Could you check a few things on this model? Use its own coordinates, in mm. Face numbers are marked on the shaded views. A direction names the side the tool comes from. Round coordinates to 2 decimals unless told otherwise and drop trailing zeros. Loops run counter-clockwise (first coordinate to the right, second up) from the corner with the lowest first, then second, coordinate; pieces in that order, holes last.
from build123d import *

# Parameters (mm, degrees)
EXTRUDE_1_DEPTH              = 2
EXTRUDE_3_DEPTH              = 6
CUT_EXTRUDE_1_REACH          = 27.426
SKETCH_5_R                   = 1.25
EXTRUDE_4_REACH              = 39.53
SKETCH_6_W                   = 10
SKETCH_6_H                   = 0.5
CUT_EXTRUDE_2_REACH          = 39.53
SKETCH_7_W                   = 8
SKETCH_7_H                   = 0.5
SKETCH_10_W                  = 1
SKETCH_10_H                  = 3.5
EXTRUDE_5_DEPTH              = 3.3
CHAMFER_1_SIZE               = 2
CUT_EXTRUDE_3_REACH          = 27.114
CUT_EXTRUDE_4_DEPTH          = 0.5
HOLE_WIZARD_M2_2_D           = 2.1
HOLE_WIZARD_M2_2_CBORE_D     = 3.8
HOLE_WIZARD_M2_2_CBORE_DEPTH = 1
FILLET_3_R                   = 2
CUT_EXTRUDE_5_DEPTH          = 0.8


with BuildPart() as part:
    # ｽｹｯﾁ1 → ﾎﾞｽ - 押し出し1 (new body)
    with BuildSketch(Plane(origin=(0, 0, 0), x_dir=(1, 0, 0), z_dir=(0, 1, 0))):
        Polygon((-13, 8), (3, 8), (13, 1), (13, -8), (-13, -8), (-13, -5), (-23.5, 2.35), (-23.5, 8), align=None)
    extrude(amount=EXTRUDE_1_DEPTH)

    # ｽｹｯﾁ4 → ﾎﾞｽ - 押し出し3 (add)
    with BuildSketch(Plane.XY.offset(8)):
        Polygon((-7, -3.5), (-4.5, -3.5), (-3, 0), (-7.9, 0), align=None)
        Polygon((3, 0), (4.5, -3.5), (7, -3.5), (7.9, 0), align=None)
    extrude(amount=-EXTRUDE_3_DEPTH)

    # ｽｹｯﾁ5 → ｶｯﾄ - 押し出し1 (cut, up to next)
    with BuildSketch(Plane(origin=(0, 2, 0), x_dir=(1, 0, 0), z_dir=(0, 1, 0)), mode=Mode.PRIVATE) as cut_extrude_1_sk1:
        with Locations(Location((0, -5, 0), (0, 0, 270))):
            Circle(SKETCH_5_R)
    cut_extrude_1_tool1 = extrude(cut_extrude_1_sk1.sketch, amount=-CUT_EXTRUDE_1_REACH, mode=Mode.PRIVATE) & part.part
    add(cut_extrude_1_tool1.solids().sort_by_distance((0, 2, 5))[0], mode=Mode.SUBTRACT)

    # ﾎﾞｽ - 押し出し4: up to this face of the body (flat: up to its plane)
    extrude_4_end = Plane(part.part.faces().sort_by_distance((-23.5, 1, -5.175))[0])
    # ｽｹｯﾁ6 → ﾎﾞｽ - 押し出し4 (add, up to the picked face)
    with BuildSketch(Plane(origin=(13, 0, 0), x_dir=(0, 0, -1), z_dir=(1, 0, 0)), mode=Mode.PRIVATE) as extrude_4_sk1:
        with Locations((3, -0.25)):
            Rectangle(SKETCH_6_W, SKETCH_6_H)
    extrude_4_tool1 = split(extrude(extrude_4_sk1.sketch, amount=-EXTRUDE_4_REACH, mode=Mode.PRIVATE), bisect_by=extrude_4_end, keep=Keep.BOTH, mode=Mode.PRIVATE)
    add(extrude_4_tool1.solids().sort_by(Axis((13, -0.25, -3), (-1, 0, 0)))[0])

    # ｽｹｯﾁ7 → ｶｯﾄ - 押し出し2 (cut, up to next)
    with BuildSketch(Plane(origin=(13, 0, 0), x_dir=(0, 0, -1), z_dir=(1, 0, 0)), mode=Mode.PRIVATE) as cut_extrude_2_sk1:
        with Locations((4, 1.75)):
            Rectangle(SKETCH_7_W, SKETCH_7_H)
    cut_extrude_2_tool1 = extrude(cut_extrude_2_sk1.sketch, amount=-CUT_EXTRUDE_2_REACH, mode=Mode.PRIVATE) & part.part
    add(cut_extrude_2_tool1.solids().sort_by_distance((13, 1.75, -4))[0], mode=Mode.SUBTRACT)

    # ｽｹｯﾁ10 → ﾎﾞｽ - 押し出し5 (add)
    with BuildSketch(Plane.XZ.offset(0.5)):
        with Locations((10.75, 0.25)):
            Rectangle(SKETCH_10_W, SKETCH_10_H)
    extrude_5 = extrude(amount=EXTRUDE_5_DEPTH)

    # ﾐﾗｰ1: ﾎﾞｽ - 押し出し5 across plane
    add(extrude_5.mirror(Plane(origin=(0, 0, 0), x_dir=(0, 0, 1), z_dir=(1, 0, 0))))

    # 面取り1
    # the kernel refuses this chamfer: 2 mm, written as the material it takes off along each edge
    with BuildSketch(Plane(origin=(18.143365976, 2, 8), x_dir=(0, -0.9996219169112968, 0.027495876610586494), z_dir=(-1, 0, 0))) as chamfer_1_piece_1:
        Polygon((CHAMFER_1_SIZE * 0.999621916911, -CHAMFER_1_SIZE * 0.0274958766106), (-CHAMFER_1_SIZE * 0.0274958766106, -CHAMFER_1_SIZE * 0.999621916911), (0, 0), align=None)
    extrude(amount=36.286731952, mode=Mode.SUBTRACT)

    # ｽｹｯﾁ12 → ｶｯﾄ - 押し出し3 (cut, up to next)
    with BuildSketch(Plane(origin=(0, 0, 0), x_dir=(1, 0, 0), z_dir=(0, 1, 0)), mode=Mode.PRIVATE) as cut_extrude_3_sk1:
        Polygon((3, 8), (13, 8), (13, 1), align=None)
    cut_extrude_3_tool1 = extrude(cut_extrude_3_sk1.sketch, amount=-CUT_EXTRUDE_3_REACH, mode=Mode.PRIVATE) & part.part
    # ｽｹｯﾁ12 → ｶｯﾄ - 押し出し3 (cut, up to next)
    with BuildSketch(Plane(origin=(0, 0, 0), x_dir=(1, 0, 0), z_dir=(0, 1, 0)), mode=Mode.PRIVATE) as cut_extrude_3_sk2:
        Polygon((-23.5, -2), (-17.285714286, -2), (-23.5, 2.35), align=None)
    cut_extrude_3_tool2 = extrude(cut_extrude_3_sk2.sketch, amount=-CUT_EXTRUDE_3_REACH, mode=Mode.PRIVATE) & part.part
    add(cut_extrude_3_tool1.solids().sort_by_distance((9.666667, 0, -5.666667))[0], mode=Mode.SUBTRACT)
    add(cut_extrude_3_tool2.solids().sort_by_distance((-21.428571, 0, 0.55))[0], mode=Mode.SUBTRACT)

    # ｽｹｯﾁ13 → ｶｯﾄ - 押し出し4 (cut)
    with BuildSketch(Plane(origin=(0, 2, 0), x_dir=(1, 0, 0), z_dir=(0, 1, 0))):
        Polygon((-13, -5), (-13, 0), (-20.142857143, 0), align=None)
    extrude(amount=-CUT_EXTRUDE_4_DEPTH, mode=Mode.SUBTRACT)

    # M2 丸平ねじ用座ぐり穴2 (through all)
    with Locations(Plane(origin=(0, 1.5, 0), x_dir=(1, 0, 0), z_dir=(0, 1, 0))):
        with Locations((-21, 4), (0, 4)):
            CounterBoreHole(HOLE_WIZARD_M2_2_D / 2, HOLE_WIZARD_M2_2_CBORE_D / 2, HOLE_WIZARD_M2_2_CBORE_DEPTH)

    # ﾌｨﾚｯﾄ3
    fillet_3_edges = [part.edges().sort_by_distance(p)[0] for p in [
        (-13, 0.75, 5),
        (13, 0.5, -1),
        (3, 0.5, -8),
        (-23.5, 0.5, -8),
        (-23.5, 0.5, -2.35),
    ]]
    fillet(fillet_3_edges, radius=FILLET_3_R)

    # ｽｹｯﾁ16 → ｶｯﾄ - 押し出し5 (cut, symmetric)
    with BuildSketch(Plane.XY.offset(5)):
        Polygon((-7.9, 0), (-7, -3.5), (-6.4, -3.5), (-7.3, 0), align=None)
        Polygon((-3, 0), (-4.5, -3.5), (-5.1, -3.5), (-3.6, 0), align=None)
        Polygon((3, 0), (4.5, -3.5), (5.1, -3.5), (3.6, 0), align=None)
        Polygon((7.9, 0), (7, -3.5), (6.4, -3.5), (7.3, 0), align=None)
    extrude(amount=CUT_EXTRUDE_5_DEPTH, both=True, mode=Mode.SUBTRACT)


solid = part.part
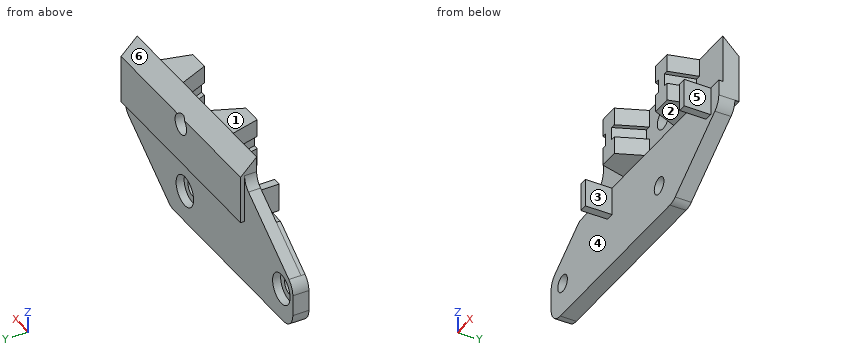
Item 1: Will these pins go through, and if not, where does the flat tip stop? pin 1 (1.1 mm diameter, centred on x = 11, y = -1, fed in from +Z); pin 2 (0.9 mm diameter, centred on x = 5.5, y = -2.5, fed in from -Z); pin 3 (8 mm diameter, centred on x = -19, z = 1.5, fed in from +Y).
Results list:
pin 1: stops at z = 2
pin 2: stops at z = 2
pin 3: stops at y = 1.5
Item 2: If we section it at B-B, the plane x = -21: Please give me the cut outline in (y, z), then the cut area to 3 significant figures.
Results list:
outline: (-0.5, -8) - (1.5, -8) - (1.5, -5.9) - (0.5, -5.9) - (0.5, -5.05) - (-0.5, -5.05) - close; (-0.5, -2.95) - (0.5, -2.95) - (0.5, -2.1) - (1.5, -2.1) - (1.5, -0.6) - (-0.5, -0.6) - close
area: 8.90 mm2
Item 3: We'd pull the mould along X, two halves only. Please class the marked faces 4, 5 and 6: released by +X, released by -X, zero draft, split by the parting line, or undercut.
Results list:
face 4: undercut
face 5: released by +X
face 6: zero draft
Item 4: If we section it at A-A, the plane y = -1.4: Count the separate pieces of the cut face and the enclosed holes in it, then the cut area to 3 significant figures.
Results list:
separate pieces: 4
enclosed holes: 0
area: 50.4 mm2
Item 5: If I drill on line 1 along Y through (x, z) = (1.5, 4.5); line 2 along Z through (x, y) = (0, -0.15); line 3 along Z through (x, y) = (-6, -1.4), over which ranges is the centre line in solid material (lowest first)?
Results list:
line 1: y = 0 to 2
line 2: z = -8 to -5.05, -2.95 to 2
line 3: z = 2 to 8
Item 6: For the marked faces 1, 2 and 3, which set-ups out of +Z, -Z, +X, -X, +Y, -Y let a thin tool reach every point of the face, with its end or its side?
Results list:
face 1: +Z, +X, -X, +Y, -Y
face 2: -Z, -Y
face 3: +Z, -Z, -Y
Item 7: If we section it at D-D, the plane z = -4.5: Please give me the cut outline in (x, y), then the cut area to 3 significant figures.
Results list:
outline: (-23.5, -0.5) - (-21.92, -0.5) - (-21.92, 0.5) - (-22.83, 0.5) - (-22.83, 1.5) - (-23.5, 1.5) - close; (-20.08, -0.5) - (-0.92, -0.5) - (-0.92, 0.5) - (-1.83, 0.5) - (-1.83, 1.5) - (-19.17, 1.5) - (-19.17, 0.5) - (-20.08, 0.5) - close; (0.92, -0.5) - (8, -0.5) - (8, 1.5) - (1.83, 1.5) - (1.83, 0.5) - (0.92, 0.5) - close
area: 52.0 mm2
Item 8: If we section it at C-C, the plane z = 5: Please give me the cut outline in (x, y), then the cut area to 3 significant figures.
Results list:
outline: (-13.29, 0) - (-7.3, 0) - (-6.4, -3.5) - (-5.1, -3.5) - (-3.6, 0) - (-1.25, 0) - (-1.25, 2) - (-13, 2) - (-13, 1.5) - (-13.29, 1.5) - close; (1.25, 0) - (3.6, 0) - (5.1, -3.5) - (6.4, -3.5) - (7.3, 0) - (13, 0) - (13, 2) - (1.25, 2) - close
area: 64.9 mm2
